Work out the finished part from the listing and answer in its coordinate system (mm). A direction names the side the tool comes from. Give positions to 0.01 mm unless a question says otherwise; leave off trailing zeros. Write each loop counter-clockwise with the first axis right and the second up, starting at its lowest first coordinate (ties: lowest second). Pieces come first, ordered by that corner, then holes.
1) Find section A-A (x = 31.75). Determine the outline of the cut face in (y, z) (3 decimals), plus the area to 3 significant figures.
2) A tool of negligible diameter and unlimited length cuts with its end or side. For faces 5 (the face through (59.06, 10.32, 1.57)), 6 (the face through (66.675, 26, 9)), from which of +Z, -Z, +X, -X, +Y, -Y can it reach the whole face along a straight path? Write none if from no direction.
3) Straight lines are drawn through the part: probe 1 along Y at (x, z) = (57.15, 1.1); probe 2 along X at (y, z) = (11, 7) (3 decimals); probe 3 along Z at (x, y) = (11, 41) (3 decimals). For each, find the intervals that lie inside material, in ascending order.
4) Find section D-D (x = 22). Determine the outline of the cut face in (y, z) (3 decimals), plus the area to 3 significant figures.
5) Find section C-C (z = 10). Determine the outline of the cut face in (x, y) (3 decimals), plus the area to 3 significant figures.
6) Given pin 1 Ø10 at (x, y) = (12.5, 6) entering from +Z (3 decimals); pin 2 Ø4 at (y, z) = (17, 8.5) entering from -X (3 decimals), each flat-ended and moving along its own axis, determine where each tip first touches the part or whether it passes through.
7) Determine the mould class of faces 1 (the face through (38, 0, 2)), 2 (the face through (31.301, 43.296, 1.565)), 3 (the face through (7.31, 11.36, 1.57)), 4 (the face through (32, 26, 3.175)) for opening direction Y: pulls with the +Y half, pulls with the -Y half, needs draft (parallel to the pull), parting line crosses it, or undercut.
8) Find section B-B (y = 46.5). Determine the outline of the cut face in (x, z) (3 decimals).
Autodesk Inventor part; units mm, degrees
ref_plane "YZ Plane" through (0, 0, 0) normal (1, 0, 0) x (0, 1, 0)
ref_plane "XZ Plane" through (0, 0, 0) normal (0, 1, 0) x (-1, 0, 0)
ref_plane "XY Plane" through (0, 0, 0) normal (0, 0, 1) x (1, 0, 0)
sketch "Sketch1" plane through (0, 0, 0) normal (0, 0, 1) x (1, 0, 0)
  line L0 (0, 0) -> (69.85, 0)
  line L1 (69.85, 0) -> (69.85, 50.8)
  line L2 (69.85, 50.8) -> (0, 50.8)
  line L3 (0, 50.8) -> (0, 0)
  circle A0 centre (6.35, 9.525) radius 2.0701
  circle A1 centre (31.75, 9.525) radius 2.0701
  circle A2 centre (57.15, 9.525) radius 2.0701
  circle A3 centre (6.35, 41.275) radius 2.0701
  circle A4 centre (31.75, 41.275) radius 2.0701
  circle A5 centre (57.15, 41.275) radius 2.0701
  dimension "d4" = 50.8
  dimension "d5" = 69.85
  dimension "d6" = 4.1402
  dimension "d7" = 6.35
  dimension "d8" = 9.525
  dimension "d9" = 25.4
  dimension "d10" = 31.75
extrude "Plate1" add sketch "Sketch1" along normal blind 3.175
sketch "Sketch2" plane through (66.675, 50.8, 0) normal (1, 0, 0) x (0, 1, 0)
  line L0 (-50.8, 0) -> (0, 0)
  line L1 (0, 0) -> (0, 12.7)
  line L2 (0, 12.7) -> (-50.8, 12.7)
  line L3 (-50.8, 12.7) -> (-50.8, 0)
edge flange "Flange1" height 12.7 angle 90 thickness 3.175 bend radius 1.27 thickness toward (1, 0, 0) relief tear relief width 3.175 relief depth 1.5875 edges at (69.85, 25.4, 3.175) wall of the first edge with corners at (66.675, 0, 0) (66.675, 50.8, 0) (66.675, 50.8, 12.7) (66.675, 0, 12.7)
bend "Bend1"
corner "Corner1"
equation "\"d12\" = BendReliefWidth"
equation "\"d13\" = BendReliefDepth"
equation "\"d14\" = MinimumRemnant"
equation "\"d15\" = BendRadius"
equation "\"d19\" = CornerReliefSize"
equation "\"d20\" = GapSize"
equation "\"d21\" = JacobiRadiusSize"
equation "\"BendRadius\" = Thickness"
equation "\"BendReliefWidth\" = Thickness"
equation "\"BendReliefDepth\" = 0.5 * Thickness"
equation "\"CornerReliefSize\" = 4 * Thickness"
equation "\"MinimumRemnant\" = 2 * Thickness"
equation "\"TransitionRadius\" = BendRadius"
equation "\"JacobiRadiusSize\" = BendRadius"
equation "\"GapSize\" = Thickness"
equation "\"d11\" = BendRadius"
properties part number "Spacer 3" material "Aluminum 6061"
Results:
1. outline: (0, 0) - (7.455, 0) - (7.455, 3.175) - (0, 3.175) - close; (11.595, 0) - (39.205, 0) - (39.205, 3.175) - (11.595, 3.175) - close; (43.345, 0) - (50.8, 0) - (50.8, 3.175) - (43.345, 3.175) - close
1. area: 135 mm2
2. face 5: +Z, -Z
2. face 6: +Z, -X, +Y, -Y
3. probe 1: y = 0 to 7.45, 11.6 to 39.2, 43.35 to 50.8
3. probe 2: x = 66.675 to 69.85
3. probe 3: z = 0 to 3.175
4. outline: (0, 0) - (50.8, 0) - (50.8, 3.175) - (0, 3.175) - close
4. area: 161 mm2
5. outline: (66.675, 0) - (69.85, 0) - (69.85, 50.8) - (66.675, 50.8) - close
5. area: 161 mm2
6. pin 1: stops at z = 3.175
6. pin 2: stops at x = 66.675
7. face 1: pulls with the -Y half
7. face 2: undercut
7. face 3: undercut
7. face 4: needs draft
8. outline: (0, 0) - (65.405, 0) arc R4.445 ccw to (69.85, 4.445) - (69.85, 12.7) - (66.675, 12.7) - (66.675, 4.445) arc R1.27 cw to (65.405, 3.175) - (0, 3.175) - close
